from build123d import *

# Parameters (mm, degrees)
F0_W     = 51.5
F0_H     = 37
F1_DEPTH = 39
F2_W     = 6
F2_H     = 21
F2_H_2   = 14
F3_DEPTH = 39.001
F4_R     = 2
F4_R_2   = 1.5
F5_DEPTH = 12
F6_R     = 2


with BuildPart() as f1:
    # F0 (on Top) → F1 (new body)
    with BuildSketch(Plane.XY):
        with Locations((25.75, 18.5)):
            Rectangle(F0_W, F0_H)
    extrude(amount=F1_DEPTH)

    # F2 (on face) → F3 (cut, through all)
    with BuildSketch(Plane(origin=(0, 0, 0), x_dir=(1, 0, 0), z_dir=(0, 0, -1))):
        with Locations((3, -10.5)):
            Rectangle(F2_W, F2_H)
        with Locations((48.5, -10.5)):
            Rectangle(F2_W, F2_H)
        with Locations((48.5, -30)):
            Rectangle(F2_W, F2_H_2)
    extrude(amount=-F3_DEPTH, mode=Mode.SUBTRACT)

    # F4 (on face) → F5 (join)
    with BuildSketch(Plane.XZ.offset(-21)):
        with Locations((48.5, 4.5)):
            Circle(F4_R)
        with Locations((48.5, 4.5)):
            Circle(F4_R_2, mode=Mode.SUBTRACT)
        with Locations((48.5, 11.5)):
            Circle(F4_R)
        with Locations((48.5, 11.5)):
            Circle(F4_R_2, mode=Mode.SUBTRACT)
        with Locations((48.5, 18.5)):
            Circle(F4_R)
        with Locations((48.5, 18.5)):
            Circle(F4_R_2, mode=Mode.SUBTRACT)
        with Locations((48.5, 25.5)):
            Circle(F4_R)
        with Locations((48.5, 25.5)):
            Circle(F4_R_2, mode=Mode.SUBTRACT)
        with Locations((48.5, 32.5)):
            Circle(F4_R)
        with Locations((48.5, 32.5)):
            Circle(F4_R_2, mode=Mode.SUBTRACT)
    extrude(amount=F5_DEPTH)

    # F6
    f6_edges = [f1.edges().sort_by_distance(p)[0] for p in [
        (0, 29, 0),
        (0, 29, 39),
    ]]
    fillet(f6_edges, radius=F6_R)


solid = f1.part
Check sheet for the modelled part. Datum: model origin and axes. Units: mm. A direction names the side the tool comes from. Round coordinates to 2 decimals unless told otherwise and drop trailing zeros. Loops run counter-clockwise (first coordinate to the right, second up) from the corner with the lowest first, then second, coordinate; pieces in that order, holes last.
1. Scan lines: probe 1 along X at (y, z) = (6.5, 25.5); probe 2 along Y at (x, z) = (47, 9.5); probe 3 along X at (y, z) = (25, 14). Record each from-to range of solid material in increasing order.
2. Sectioned sample at B-B on y = 25. Record the boundary of the cut face in (x, z), and give its area (3 significant figures).
3. Gauge pin test, flat ends, axial feed: pin 1 Ø4 at (x, z) = (48.5, 11.5) entering from +Y; pin 2 Ø12 at (y, z) = (9, 14.5) entering from +X; pin 3 Ø3.5 at (x, z) = (49, 11) entering from -Y; pin 4 Ø6.5 at (x, z) = (3, 13) entering from -Y. Record the tip position at first contact, or that the pin passes through.
4. Sectioned sample at A-A on z = 7.5. Record the boundary of the cut face in (x, y), and give its area (3 significant figures).
5. Set-up check for faces 1 (the flat face through (45.5, 11, 19)), 2 (the flat face through (45.5, 30, 19)), 3 (the cylindrical face through (46.502, 15.084, 4.588)): record each of +Z, -Z, +X, -X, +Y, -Y from which the full face is reachable in a straight line by a thin tool's end or side.
6. Sectioned sample at C-C on z = 32.5. Record the boundary of the cut face in (x, y), and give its area (3 significant figures).
7. Mould release check, pull along X, two halves, no side actions. Record for faces 4 (the cylindrical face through (48.24, 15.084, 13.483)), 5 (the cylindrical face through (48.066, 15.084, 23.548)), 6 (the flat face through (6, 11, 19)), 7 (the flat face through (26, 19, 0)): released by +X, released by -X, zero draft, split by the parting line, or undercut.
8. Sectioned sample at D-D on x = 4. Record the boundary of the cut face in (y, z).
Recorded:
1. probe 1: x = 6 to 45.5
1. probe 2: y = 21 to 23
1. probe 3: x = 0 to 45.5
2. outline: (0, 2) arc R2 ccw to (2, 0) - (45.5, 0) - (45.5, 39) - (2, 39) arc R2 ccw to (0, 37) - close
2. area: 1,770 mm2
3. pin 1: stops at y = 23
3. pin 2: stops at x = 50.5
3. pin 3: stops at y = 9
3. pin 4: stops at y = 0
4. outline: (0, 21) - (6, 21) - (6, 0) - (45.5, 0) - (45.5, 21) - (51.5, 21) - (51.5, 23) - (45.5, 23) - (45.5, 37) - (0, 37) - close
4. area: 1,570 mm2
5. face 1: +Z, -Z, -Y
5. face 2: +Z, -Z, +X, +Y
5. face 3: -Y
6. outline: (0, 21) - (6, 21) - (6, 0) - (45.5, 0) - (45.5, 21) - (46.5, 21) - (46.5, 9) - (47, 9) - (47, 21) - (50, 21) - (50, 9) - (50.5, 9) - (50.5, 21) - (51.5, 21) - (51.5, 23) - (45.5, 23) - (45.5, 37) - (0, 37) - close
6. area: 1,580 mm2
7. face 4: undercut
7. face 5: undercut
7. face 6: released by -X
7. face 7: zero draft
8. outline: (21, 0) - (37, 0) - (37, 39) - (21, 39) - close
